```python
from build123d import *

# Parameters (mm, degrees)
SKETCH1_W           = 200
SKETCH1_H           = 15.875
SKETCH1_W_2         = 15.875
SKETCH1_H_2         = 60
BOSS_EXTRUDE1_DEPTH = 15.875
SKETCH2_R           = 4
CUT_EXTRUDE1_DEPTH  = 16.875


with BuildPart() as part:
    # Sketch1 → Boss-Extrude1 (new body)
    with BuildSketch(Plane(origin=(0, 0, 0), x_dir=(0, 0, -1), z_dir=(1, 0, 0))):
        Rectangle(SKETCH1_W, SKETCH1_H)
        with Locations((0, 37.9375)):
            Rectangle(SKETCH1_W_2, SKETCH1_H_2)
    extrude(amount=BOSS_EXTRUDE1_DEPTH)

    # Sketch2 → Cut-Extrude1 (cut, through all)
    with BuildSketch(Plane(origin=(15.875, 0, 0), x_dir=(0, 0, -1), z_dir=(1, 0, 0))):
        with Locations((0, 57.9375)):
            Circle(SKETCH2_R)
    extrude(amount=-CUT_EXTRUDE1_DEPTH, mode=Mode.SUBTRACT)


solid = part.part
```
Read the model definition and answer for the solid it produces. Units are mm, in the model's axes. A direction names the side the tool comes from. Coordinates: 2 decimals unless noted, no trailing zeros. Order: outer loops, then holes, each group sorted by start corner. A loop starts at its lowest first (then second) coordinate and runs counter-clockwise, first axis right, second up. Notation, with made-up numbers: (18, 51.5) - (49, 51.5) arc R17 cw to (49, 71.5) - close; hole circle Ø10 at (7.25, -23.75). An arc over 180 degrees is marked (long way). Answer as a JSON object with one key per item and string values. Group by question number.
Item 1: Flat-ended cylindrical pins translate along their axes: P1, Ø8, axis at x = 7, z = 37, coming from the +Y side; P2, Ø1, axis at y = 7.5, z = -30, coming from the -X side; P3, Ø5, axis at x = 8, y = 33, coming from the +Z side. Find the tip coordinate at first contact, or state that the pin passes through.
Item 2: Consider probe 1 along Y at (x, z) = (8.5, 0); probe 2 along Z at (x, y) = (6.75, 20.5). Determine where each line is inside the solid, lowest interval first. Write a range as from..to.
Item 3: Section B-B (x = 11.5) is taken. Give the vertices of the cut face in (y, z).
Item 4: The mould has two halves that part along Y. Classify faces 3 (the face through (8, -7.938, 1)), 4 (the face through (8, 7.938, -53)), 5 (the face through (8.049, 54.033, 0.867)), 6 (the face through (8, 38, -7.938)): +Y half, -Y half, draft (parallel to the pull), parting line (faces both ways), or undercut.
Item 5: A tool of negligible diameter and unlimited length cuts with its end or side. For faces 1 (the face through (15.875, 8, 0)), 2 (the face through (8, 38, 7.938)), from which of +Z, -Z, +X, -X, +Y, -Y can it reach the whole face along a straight path? Write none if from no direction.
Item 6: Section C-C (y = 16.5) is taken. Give the vertices of the cut face in (x, z) (1 decimal).
Item 7: Section A-A (z = 0) is taken. Give the vertices of the cut face in (x, y) (1 decimal).
Results are:
{
 "1": {"P1": "stops at y = 7.94", "P2": "stops at x = 0", "P3": "stops at z = 7.94"},
 "2": {"probe 1": "y = -7.94..53.94, 61.94..67.94", "probe 2": "z = -7.94..7.94"},
 "3": {"outline": "(-7.94, -100) - (7.94, -100) - (7.94, -7.94) - (67.94, -7.94) - (67.94, 7.94) - (7.94, 7.94) - (7.94, 100) - (-7.94, 100) - close; hole circle Ø8 at (57.94, 0)"},
 "4": {"face 3": "-Y half", "face 4": "+Y half", "face 5": "undercut", "face 6": "draft"},
 "5": {"face 1": "+Z, -Z, +X, +Y, -Y", "face 2": "+Z, +X, -X, +Y"},
 "6": {"outline": "(0, -7.9) - (15.9, -7.9) - (15.9, 7.9) - (0, 7.9) - close"},
 "7": {"outline": "(0, -7.9) - (15.9, -7.9) - (15.9, 53.9) - (0, 53.9) - close; (0, 61.9) - (15.9, 61.9) - (15.9, 67.9) - (0, 67.9) - close"}
}
